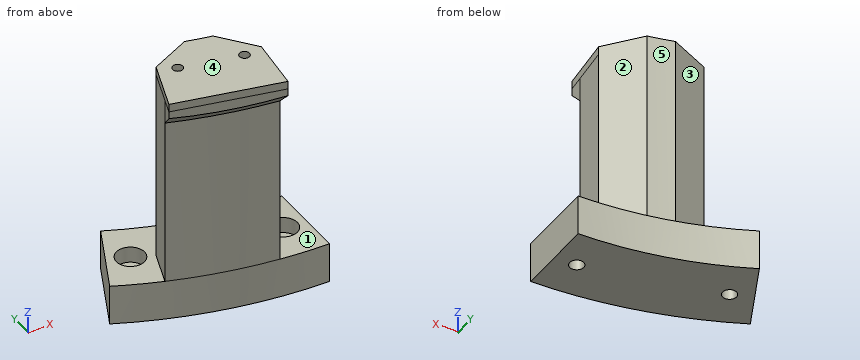
from build123d import *

# Parameters (mm, degrees)
BOSS_EXTRU_1_DEPTH      = 10
BOSS_EXTRU_2_DEPTH      = 48
BOSS_EXTRU_3_DEPTH      = 2
CHANFREIN1_SIZE         = 6
ENL_V_MAT_EXTRU_1_REACH = 138.536
ESQUISSE5_R             = 1.75
ESQUISSE6_R             = 3.5
ENL_V_MAT_EXTRU_2_DEPTH = 4
CHANFREIN2_SIZE         = 7.5
ESQUISSE7_R             = 1.25
ENL_V_MAT_EXTRU_3_DEPTH = 10


with BuildPart() as part:
    # Esquisse1 → Boss.-Extru.1 (new body)
    with BuildSketch(Plane.XY):
        with BuildLine():
            Line((-39.726116604, -85.192931981), (-48.178481838, -103.319087722))
            ThreePointArc((-48.178481838, -103.319087722), (-24.674115989, -111.297744812), (0, -114))
            Line((0, -114), (0, -94))
            ThreePointArc((0, -94), (-20.34532371, -91.771824669), (-39.726116604, -85.192931981))
        make_face()
    extrude(amount=BOSS_EXTRU_1_DEPTH)

    # Esquisse2 → Boss.-Extru.2 (add)
    with BuildSketch(Plane.XY.offset(10)):
        with BuildLine():
            Line((-31.580110982, -91.715301833), (-37.114769608, -107.789117618))
            ThreePointArc((-37.114769608, -107.789117618), (-24.674115989, -111.297744812), (-11.916244813, -113.375496072))
            Line((-11.916244813, -113.375496072), (-10.139260937, -96.468623851))
            ThreePointArc((-10.139260937, -96.468623851), (-20.994642552, -94.700712691), (-31.580110982, -91.715301833))
        make_face()
    extrude(amount=BOSS_EXTRU_2_DEPTH)

    # Esquisse4 → Boss.-Extru.3 (add)
    with BuildSketch(Plane.XY.offset(58)):
        with BuildLine():
            Line((-38.485369249, -111.769628004), (-12.356296065, -117.562304069))
            Line((-12.356296065, -117.562304069), (-10.139260937, -96.468623851))
            ThreePointArc((-10.139260937, -96.468623851), (-20.994642552, -94.700712691), (-31.580110982, -91.715301833))
            Line((-31.580110982, -91.715301833), (-38.485369249, -111.769628004))
        make_face()
    extrude(amount=BOSS_EXTRU_3_DEPTH)

    # Chanfrein1
    # the kernel refuses this chamfer: 6 mm, written as the material it adds along each edge
    with BuildSketch(Plane(origin=(0, 0, 58), x_dir=(-0.3255681544571537, -0.9455185755993178, 0), z_dir=(-0.9455185755993178, 0.3255681544571537, 0))) as chanfrein1_piece_1_section:
        Polygon((114 + CHANFREIN1_SIZE, 0), (114, -CHANFREIN1_SIZE), (114, 0), align=None)
    chanfrein1_piece_1 = revolve(axis=Axis((0, 0, 58), (0, 0, 1)), revolution_arc=13, mode=Mode.PRIVATE)
    chanfrein1_piece_1 = split(chanfrein1_piece_1, bisect_by=Plane(origin=(-25.420832657, -114.665966036, 58), z_dir=(0.21643961393810382, 0.9762960071199333, 0)), keep=Keep.TOP, mode=Mode.PRIVATE)
    add(chanfrein1_piece_1)

    # Esquisse5 → Enlèv. mat.-Extru.1 (cut, up to next)
    with BuildSketch(Plane.XY.offset(10), mode=Mode.PRIVATE) as enl_v_mat_extru_1_sk1:
        with Locations((-5.442939449, -103.857471614)):
            Circle(ESQUISSE5_R)
    enl_v_mat_extru_1_tool1 = extrude(enl_v_mat_extru_1_sk1.sketch, amount=-ENL_V_MAT_EXTRU_1_REACH, mode=Mode.PRIVATE) & part.part
    # Esquisse5 → Enlèv. mat.-Extru.1 (cut, up to next)
    with BuildSketch(Plane.XY.offset(10), mode=Mode.PRIVATE) as enl_v_mat_extru_1_sk2:
        with Locations((-38.959085715, -96.427120875)):
            Circle(ESQUISSE5_R)
    enl_v_mat_extru_1_tool2 = extrude(enl_v_mat_extru_1_sk2.sketch, amount=-ENL_V_MAT_EXTRU_1_REACH, mode=Mode.PRIVATE) & part.part
    add(enl_v_mat_extru_1_tool1.solids().sort_by_distance((-5.442939, -103.857472, 10))[0], mode=Mode.SUBTRACT)
    add(enl_v_mat_extru_1_tool2.solids().sort_by_distance((-38.959086, -96.427121, 10))[0], mode=Mode.SUBTRACT)

    # Esquisse6 → Enlèv. mat.-Extru.2 (cut)
    with BuildSketch(Plane.XY.offset(10)):
        with Locations((-38.959085715, -96.427120875)):
            Circle(ESQUISSE6_R)
        with Locations((-5.442939449, -103.857471614)):
            Circle(ESQUISSE6_R)
    extrude(amount=-ENL_V_MAT_EXTRU_2_DEPTH, mode=Mode.SUBTRACT)

    # Chanfrein2
    # the kernel refuses this chamfer: 7.5 mm, written as the material it takes off along each edge
    with BuildSketch(Plane(origin=(-10.139260937, -96.468623851, 10), x_dir=(-0.10452846326693861, -0.9945218953683486, 0), z_dir=(0, 0, 1)), Plane(origin=(-31.580110982, -91.715301833, 80.112002728), x_dir=(-0.3255681544565627, -0.9455185755995213, 0), z_dir=(0, 0, -1))) as chanfrein2_piece_1:
        with BuildLine():
            Line((CHANFREIN2_SIZE, 0), (-0.315356984, -7.815356984))
            ThreePointArc((-0.315356984, -7.815356984), (-0.083387766, -4.021227803), (0, 0))
            Line((0, 0), (CHANFREIN2_SIZE, 0))
        make_face()
    extrude(amount=70.112002728, mode=Mode.SUBTRACT)

    # Esquisse7 → Enlèv. mat.-Extru.3 (cut)
    with BuildSketch(Plane.XY.offset(60)):
        with Locations((-30.156599324, -101.375931647)):
            Circle(ESQUISSE7_R)
        with Locations((-15.512159217, -104.622525856)):
            Circle(ESQUISSE7_R)
    extrude(amount=-ENL_V_MAT_EXTRU_3_DEPTH, mode=Mode.SUBTRACT)


solid = part.part
Can you work these out from the model? Positions are in its coordinate system, mm. Face numbers are marked on the shaded views. A direction names the side the tool comes from. Coordinates: 2 decimals unless noted, no trailing zeros. Write each loop counter-clockwise with the first axis right and the second up, starting at its lowest first coordinate (ties: lowest second). Pieces come first, ordered by that corner, then holes. Notation, with made-up numbers: (10, 54) -> (22, 54) arc R28 cw to (22, 85) -> close; hole circle Ø1 at (-25.75, 80.5). An arc over 180 degrees is marked (long way). Write each question's results on one line, items separated by ' | '. Start each with the question number.
Q1. On a 3-axis mill with a long thin cutter (end or side, diameter ignored), from which of +Z, -Z, +X, -X, +Y, -Y can I reach the whole of each face in a straight line? I mean the marked faces 4 and 5. Say none if no direction works.
Q2. If I drill on probe 1 along Z at (x, y) = (-16.5, -104); probe 2 along Z at (x, y) = (-38, -106); probe 3 along X at (y, z) = (-96.5, 3), over which ranges is the centre line in solid material (lowest first)?
Q3. We'd pull the mould along X, two halves only. Please class the marked faces 1, 2 and 3: +X half, -X half, draft (parallel to the pull), parting line (faces both ways), or undercut.
Q4. Imagine slicing it at C-C (x = -10). Write out the boundary of the cut face in (y, z).
Q5. Imagine slicing it at A-A (z = 7.5). Write out the boundary of the cut face in (x, y), then the cut area to 3 significant figures.
Q6. I'm going to push flat-ended pins straight in: pin 1 (2 mm diameter, centred on x = -30, y = -101, fed in from +Z); pin 2 (1.5 mm diameter, centred on x = -14, z = 20, fed in from -Y); pin 3 (8 mm diameter, centred on x = -12.5, z = 43, fed in from -Y); pin 4 (9 mm diameter, centred on x = -38.96, y = -96.43, fed in from +Z). Where does each tip first touch, or does it pass through?
Q7. Imagine slicing it at B-B (z = 21.5). Write out the boundary of the cut face in (x, y), then the cut area to 3 significant figures.
Taken from the geometry:
1) face 4: +Z, +X, -X, +Y, -Y | face 5: +Z, +X, +Y
2) probe 1: z = 0 to 50 | probe 2: z = 0 to 10 | probe 3: x = -45 to -40.71, -37.21 to 0
3) face 1: draft | face 2: +X half | face 3: -X half
4) outline: (-113.56, 0) -> (-93.47, 0) -> (-93.47, 10) -> (-113.56, 10) -> close
5) outline: (-48.18, -103.32) arc R114 ccw to (0, -114) -> (0, -94) arc R94 cw to (-39.73, -85.19) -> close; hole circle Ø7 at (-38.96, -96.43); hole circle Ø7 at (-5.44, -103.86) | area: 831 mm^2
6) pin 1: stops at z = 60 | pin 2: stops at y = -113.23 | pin 3: stops at y = -113.38 | pin 4: stops at z = 10
7) outline: (-37.11, -107.79) arc R114 ccw to (-11.92, -113.38) -> (-10.92, -103.93) -> (-17.88, -95.34) arc R97 cw to (-24.09, -93.96) -> (-34.02, -98.81) -> close | area: 349 mm^2
